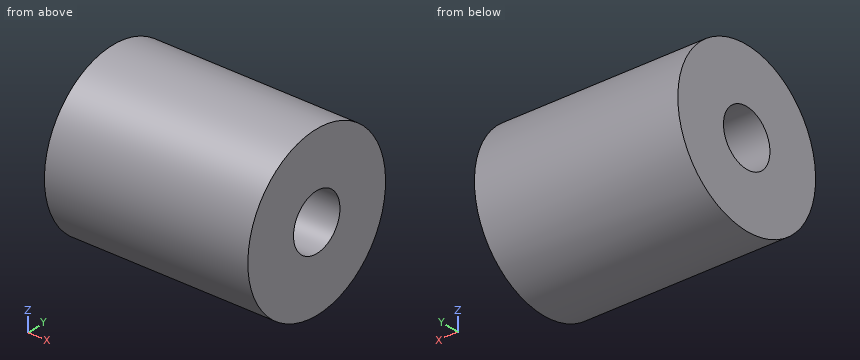
```python
from build123d import *

# Parameters (mm, degrees)
EXTRUDE1_START              = -15.4
SKETCH1_R                   = 12.5
EXTRUDE1_DEPTH              = 30.8
F_3_8_24_TAPPED_HOLE3_D     = 8.4328
F_3_8_24_TAPPED_HOLE3_DEPTH = 15
F_3_8_24_TAPPED_HOLE3_TIP   = 2.533468714
F_3_8_24_TAPPED_HOLE4_D     = 8.4328
F_3_8_24_TAPPED_HOLE4_DEPTH = 18
F_3_8_24_TAPPED_HOLE4_TIP   = 2.533468714


with BuildPart() as part:
    # Sketch1 → Extrude1 (new body)
    with BuildSketch(Plane(origin=(0, 0, 0), x_dir=(0, 0, -1), z_dir=(1, 0, 0)).offset(EXTRUDE1_START)):
        Circle(SKETCH1_R)
    extrude(amount=EXTRUDE1_DEPTH)

    # 3_8-24 Tapped Hole3
    with Locations(Plane.ZY.offset(15.4)):
        with Locations((0, 0)):
            Hole(F_3_8_24_TAPPED_HOLE3_D / 2, depth=F_3_8_24_TAPPED_HOLE3_DEPTH)
            with Locations((0, 0, -(F_3_8_24_TAPPED_HOLE3_DEPTH + F_3_8_24_TAPPED_HOLE3_TIP / 2))):  # 118° drill point
                Cone(0, F_3_8_24_TAPPED_HOLE3_D / 2, F_3_8_24_TAPPED_HOLE3_TIP, mode=Mode.SUBTRACT)

    # 3_8-24 Tapped Hole4
    with Locations(Plane(origin=(15.4, 0, 0), x_dir=(0, 0, -1), z_dir=(1, 0, 0))):
        with Locations((0, 0)):
            Hole(F_3_8_24_TAPPED_HOLE4_D / 2, depth=F_3_8_24_TAPPED_HOLE4_DEPTH)
            with Locations((0, 0, -(F_3_8_24_TAPPED_HOLE4_DEPTH + F_3_8_24_TAPPED_HOLE4_TIP / 2))):  # 118° drill point
                Cone(0, F_3_8_24_TAPPED_HOLE4_D / 2, F_3_8_24_TAPPED_HOLE4_TIP, mode=Mode.SUBTRACT)


solid = part.part
```
Model file for the job. Use its own axes, mm. Coordinates: 2 decimals unless noted, no trailing zeros. Order: outer loops, then holes, each group sorted by start corner. A loop starts at its lowest first (then second) coordinate and runs counter-clockwise, first axis right, second up. Notation, with made-up numbers: (-6.5, -40) -> (3.5, -40) arc R12 cw to (3.5, -36) -> close; hole circle Ø9 at (88.5, 21). An arc over 180 degrees is marked (long way). Answer as a JSON object with one key per item and string values. Group by question number.
1) Flat gauge pins, fed straight in: pin 1 (2 mm diameter, centred on x = 5, y = -9.5, fed in from -Z); pin 2 (1 mm diameter, centred on x = -5.5, z = -4, fed in from +Y); pin 3 (1.5 mm diameter, centred on x = -7.5, z = -4.5, fed in from -Y). Where does each tip first touch, or does it go through?
2) Cut at C-C, the plane x = -10. Write the cut outline in (y, z).
3) Drill centre lines: L1, parallel to Y at x = 11.5, z = 0; L2, parallel to Y at x = 2, z = 1.25; L3, parallel to Z at x = 13, y = -1.75. Where is each one in solid material? Low to high.
4) Cut at B-B, the plane y = 3.25. Write the cut outline in (x, z), then the cut area to 3 significant figures.
5) Cut at A-A, the plane z = 0. Write the cut outline in (x, y), then the cut area to 3 significant figures.
6) Cut at D-D, the plane z = -7.75. Write the cut outline in (x, y), then the cut area to 3 significant figures.
Check values:
{
 "1": {"pin 1": "stops at z = -9.17", "pin 2": "stops at y = 12", "pin 3": "stops at y = -11.92"},
 "2": {"outline": "circle Ø25 at (0, 0); hole circle Ø8.43 at (0, 0)"},
 "3": {"L1": "y = -12.5 to -4.22, 4.22 to 12.5", "L2": "y = -12.44 to -4.03, 4.03 to 12.44", "L3": "z = -12.38 to -3.84, 3.84 to 12.38"},
 "4": {"outline": "(-15.4, -12.07) -> (15.4, -12.07) -> (15.4, -2.69) -> (-15.4, -2.69) -> close; (-15.4, 2.69) -> (15.4, 2.69) -> (15.4, 12.07) -> (-15.4, 12.07) -> close", "area": "578 mm²"},
 "5": {"outline": "(-15.4, -12.5) -> (15.4, -12.5) -> (15.4, -4.22) -> (-15.4, -4.22) -> close; (-15.4, 4.22) -> (15.4, 4.22) -> (15.4, 12.5) -> (-15.4, 12.5) -> close", "area": "510 mm²"},
 "6": {"outline": "(-15.4, -9.81) -> (15.4, -9.81) -> (15.4, 9.81) -> (-15.4, 9.81) -> close", "area": "604 mm²"}
}
